```python
from build123d import *


with BuildPart() as part:
    # Sketch2 → Revolve1 (revolve)
    with BuildSketch(Plane.XY, mode=Mode.PRIVATE) as revolve1_sk:
        Polygon((-7.75, 11), (0, 11), (0, 20), (-7.75, 20), (-7.75, 14), align=None)
        Polygon((-7.75, 14), (-7.75, 20), (-7.75, 22), (-10.75, 22), align=None)
        Polygon((0, 20), (0, 11), (7.75, 11), (7.75, 14), (7.75, 20), align=None)
        Polygon((7.75, 22), (7.75, 20), (7.75, 14), (10.75, 22), align=None)
    revolve(revolve1_sk.sketch.rotate(Axis((11.825, 0, 0), (-1, 0, 0)), 90), axis=Axis((11.825, 0, 0), (-1, 0, 0)))


solid = part.part
```
Read the model definition and answer for the solid it produces. Units are mm, in the model's axes. A direction names the side the tool comes from. Give positions to 0.01 mm unless a question says otherwise; leave off trailing zeros. Loops run counter-clockwise (first coordinate to the right, second up) from the corner with the lowest first, then second, coordinate; pieces in that order, holes last.
Item 1: The part is cut by section C-C (x = 1.5). Write down the section's boundary in (y, z).
Item 2: The part is cut by section A-A (y = 0). Write down the section's boundary in (x, z), and give its area (3 significant figures).
Item 3: Find the intervals of material crossed by line 1 along Y through (x, z) = (-3.75, 0); line 2 along X through (y, z) = (10, -6); line 3 along Z through (x, y) = (7.25, 4), in increasing order.
Item 4: Each of these flat-tipped pins is pushed along its axis until it touches: pin 1 Ø14 at (y, z) = (2, 2.5) entering from +X; pin 2 Ø6 at (x, z) = (-0.5, -10.5) entering from +Y; pin 3 Ø5 at (x, y) = (-4.5, -16) entering from -Z; pin 4 Ø14 at (y, z) = (3, 5.5) entering from -X. Where does it stop, or does it pass through?
Item 5: The part is cut by section D-D (x = -8.75). Write down the section's boundary in (y, z).
Item 6: The mould has two halves that part along Z. Classify faces 1 (the conical face through (-7.896, -0.633, 14.375)), 2 (the cylindrical face through (-9.271, 21.477, 4.769)), 3 (the flat face through (-7.75, 18, 10)): released by +Z, released by -Z, zero draft, split by the parting line, or undercut.
Item 7: For faces 4 (the flat face through (7.75, 18, -10)), 5 (the flat face through (-7.75, 9.3, -6.2)), 6 (the flat face through (7.75, 9.3, 6.2)), determine the directions among +Z, -Z, +X, -X, +Y, -Y from which every point of the face is accessible in a straight line to the end or side of a thin tool.
Taken from the geometry:
1. outline: circle Ø40 at (0, 0); hole circle Ø22 at (0, 0)
2. outline: (-10.75, -22) - (-7.75, -22) - (-7.75, -20) - (7.75, -20) - (7.75, -22) - (10.75, -22) - (7.75, -14) - (7.75, -11) - (-7.75, -11) - (-7.75, -14) - close; (-10.75, 22) - (-7.75, 14) - (-7.75, 11) - (7.75, 11) - (7.75, 14) - (10.75, 22) - (7.75, 22) - (7.75, 20) - (-7.75, 20) - (-7.75, 22) - close
2. area: 327 mm2
3. line 1: y = -20 to -11, 11 to 20
3. line 2: x = -7.75 to 7.75
3. line 3: z = -19.6 to -10.25, 10.25 to 19.6
4. pin 1: passes through
4. pin 2: stops at y = 18.54
4. pin 3: stops at z = -14.76
4. pin 4: stops at x = -7.75
5. outline: circle Ø44 at (0, 0); hole circle Ø33.33 at (0, 0)
6. face 1: undercut
6. face 2: split by the parting line
6. face 3: zero draft
7. face 4: none
7. face 5: -X
7. face 6: +X
